Study the drawing (mm; zero at the part's minimum x, y, z) and answer. A direction names the side the tool comes from. Coordinates: 2 decimals unless noted, no trailing zeros. Order: outer loops, then holes, each group sorted by start corner. A loop starts at its lowest first (then second) coordinate and runs counter-clockwise, first axis right, second up.
1. The part is cut by section C-C, the plane x = 12. Give the vertices of the cut face in (y, z), then the cut area to 3 significant figures.
2. The part is cut by section A-A, the plane z = 25. Give the vertices of the cut face in (x, y), then the cut area to 3 significant figures.
3. Find the intervals of material crossed by probe 1 along Y at (x, z) = (11.5, 26.5); probe 2 along X at (y, z) = (27.5, 18); probe 3 along Z at (x, y) = (23.5, 44.5), in increasing order.
4. Determine the mould class of the marked faces 4, 5, 6 and 7 for opening direction Y: +Y half, -Y half, draft (parallel to the pull), parting line (faces both ways), or undercut.
5. The part is cut by section B-B, the plane y = 28. Give the vertices of the cut face in (x, z).
6. A tool of negligible diameter and unlimited length cuts with its end or side. For the marked faces 1, 2 and 3, from which of +Z, -Z, +X, -X, +Y, -Y can it reach the whole face along a straight path? Write none if from no direction.
7. Flat-ended cylindrical pins translate along their axes: pin 1 Ø12 at (x, y) = (39, 33.5) entering from +Z; pin 2 Ø15 at (x, y) = (11.5, 53.5) entering from +Z; pin 3 Ø7 at (x, z) = (14, 26) entering from -Y. Find the tip coordinate at first contact, or state that the pin passes through.
8. The part is cut by section D-D, the plane z = 12.5. Give the vertices of the cut face in (x, y), then the cut area to 3 significant figures.
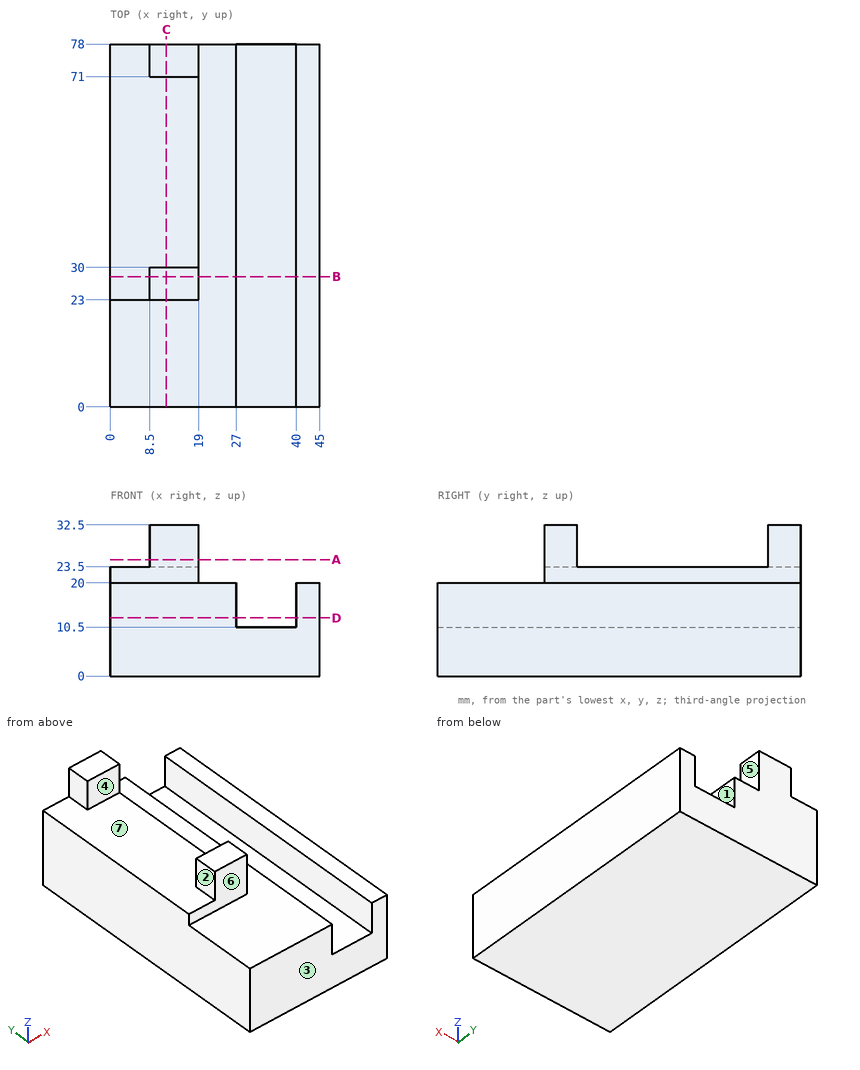
Geometry says:
1. outline: (0, 0) - (78, 0) - (78, 32.5) - (71, 32.5) - (71, 23.5) - (30, 23.5) - (30, 32.5) - (23, 32.5) - (23, 20) - (0, 20) - close
1. area: 1,880 mm2
2. outline: (8.5, 23) - (19, 23) - (19, 30) - (8.5, 30) - close; (8.5, 71) - (19, 71) - (19, 78) - (8.5, 78) - close
2. area: 147 mm2
3. probe 1: y = 23 to 30, 71 to 78
3. probe 2: x = 0 to 27, 40 to 45
3. probe 3: z = 0 to 20
4. face 4: undercut
4. face 5: draft
4. face 6: -Y half
4. face 7: undercut
5. outline: (0, 0) - (45, 0) - (45, 20) - (40, 20) - (40, 10.5) - (27, 10.5) - (27, 20) - (19, 20) - (19, 32.5) - (8.5, 32.5) - (8.5, 23.5) - (0, 23.5) - close
6. face 1: +Z, +Y, -Y
6. face 2: +Z, -X, +Y, -Y
6. face 3: +Z, -Z, +X, -X, -Y
7. pin 1: stops at z = 20
7. pin 2: stops at z = 23.5
7. pin 3: stops at y = 23
8. outline: (0, 0) - (27, 0) - (27, 78) - (0, 78) - close; (40, 0) - (45, 0) - (45, 78) - (40, 78) - close
8. area: 2,500 mm2
